```python
from build123d import *

# Parameters (mm, degrees)
SKETCH1_R           = 15
BOSS_EXTRUDE1_DEPTH = 8
BOSS_EXTRUDE2_START = 3
SKETCH2_R           = 16
BOSS_EXTRUDE2_DEPTH = 2
BOSS_EXTRUDE3_START = 3
SKETCH3_R           = 13.5
BOSS_EXTRUDE3_DEPTH = 2
BOSS_EXTRUDE4_START = -1
SKETCH4_R           = 3.6
BOSS_EXTRUDE4_DEPTH = 10
BOSS_EXTRUDE5_START = -1
SKETCH5_R           = 0.9
BOSS_EXTRUDE5_DEPTH = 10
BOSS_EXTRUDE6_START = -1
SKETCH6_R           = 0.9
BOSS_EXTRUDE6_DEPTH = 10
BOSS_EXTRUDE7_START = -1
SKETCH7_R           = 0.9
BOSS_EXTRUDE7_DEPTH = 10
BOSS_EXTRUDE8_START = -1
SKETCH8_R           = 0.9
BOSS_EXTRUDE8_DEPTH = 10


with BuildPart() as part:
    # Sketch1 → Boss-Extrude1 (new body)
    with BuildSketch(Plane(origin=(0, 0, 0), x_dir=(0, 0, -1), z_dir=(1, 0, 0))):
        Circle(SKETCH1_R)
    extrude(amount=BOSS_EXTRUDE1_DEPTH)


with BuildPart() as body_2:
    # Sketch2 → Boss-Extrude2 (new body)
    with BuildSketch(Plane(origin=(0, 0, 0), x_dir=(0, 0, -1), z_dir=(1, 0, 0)).offset(BOSS_EXTRUDE2_START)):
        Circle(SKETCH2_R)
    extrude(amount=BOSS_EXTRUDE2_DEPTH)


with BuildPart() as part_1:
    add(part.part)

    # Combine1: cut body 2
    add(body_2.part, mode=Mode.SUBTRACT)

    # Sketch3 → Boss-Extrude3 (add)
    with BuildSketch(Plane(origin=(0, 0, 0), x_dir=(0, 0, -1), z_dir=(1, 0, 0)).offset(BOSS_EXTRUDE3_START)):
        Circle(SKETCH3_R)
    extrude(amount=BOSS_EXTRUDE3_DEPTH)


with BuildPart() as body_2_2:
    # Sketch4 → Boss-Extrude4 (new body)
    with BuildSketch(Plane(origin=(0, 0, 0), x_dir=(0, 0, -1), z_dir=(1, 0, 0)).offset(BOSS_EXTRUDE4_START)):
        Circle(SKETCH4_R)
    extrude(amount=BOSS_EXTRUDE4_DEPTH)


with BuildPart() as part_2:
    add(part_1.part)

    # Combine2: cut body 2 2
    add(body_2_2.part, mode=Mode.SUBTRACT)


with BuildPart() as body_2_3:
    # Sketch5 → Boss-Extrude5 (new body)
    with BuildSketch(Plane(origin=(0, 0, 0), x_dir=(0, 0, -1), z_dir=(1, 0, 0)).offset(BOSS_EXTRUDE5_START)):
        with Locations((0, -10)):
            Circle(SKETCH5_R)
    extrude(amount=BOSS_EXTRUDE5_DEPTH)


with BuildPart() as part_3:
    add(part_2.part)

    # Combine3: cut body 2 3
    add(body_2_3.part, mode=Mode.SUBTRACT)


with BuildPart() as body_2_4:
    # Sketch6 → Boss-Extrude6 (new body)
    with BuildSketch(Plane(origin=(0, 0, 0), x_dir=(0, 0, -1), z_dir=(1, 0, 0)).offset(BOSS_EXTRUDE6_START)):
        with Locations((0, -7)):
            Circle(SKETCH6_R)
    extrude(amount=BOSS_EXTRUDE6_DEPTH)


with BuildPart() as part_4:
    add(part_3.part)

    # Combine4: cut body 2 4
    add(body_2_4.part, mode=Mode.SUBTRACT)


with BuildPart() as body_2_5:
    # Sketch7 → Boss-Extrude7 (new body)
    with BuildSketch(Plane(origin=(0, 0, 0), x_dir=(0, 0, -1), z_dir=(1, 0, 0)).offset(BOSS_EXTRUDE7_START)):
        with Locations((0, 7)):
            Circle(SKETCH7_R)
    extrude(amount=BOSS_EXTRUDE7_DEPTH)


with BuildPart() as part_5:
    add(part_4.part)

    # Combine5: cut body 2 5
    add(body_2_5.part, mode=Mode.SUBTRACT)


with BuildPart() as body_2_6:
    # Sketch8 → Boss-Extrude8 (new body)
    with BuildSketch(Plane(origin=(0, 0, 0), x_dir=(0, 0, -1), z_dir=(1, 0, 0)).offset(BOSS_EXTRUDE8_START)):
        with Locations((0, 10)):
            Circle(SKETCH8_R)
    extrude(amount=BOSS_EXTRUDE8_DEPTH)


with BuildPart() as part_6:
    add(part_5.part)

    # Combine6: cut body 2 6
    add(body_2_6.part, mode=Mode.SUBTRACT)


solid = part_6.part
```
Input: part model. Units: mm. Frame: model coordinates. A direction names the side the tool comes from. Round coordinates to 2 decimals unless told otherwise and drop trailing zeros. Loops run counter-clockwise (first coordinate to the right, second up) from the corner with the lowest first, then second, coordinate; pieces in that order, holes last. Notation, with made-up numbers: (80, 31) -> (101, 31) arc R10 cw to (101, 38) -> close; hole circle Ø9 at (56.25, -25). An arc over 180 degrees is marked (long way). Use one line per item in the form item = value. Start each with the question number.
Item 1: Contact query for flat-ended pins moving along their axis: pin 1 Ø3 at (x, y) = (4, 10.5) entering from -Z; pin 2 Ø2 at (x, z) = (5.5, -7.5) entering from +Y; pin 3 Ø2 at (x, z) = (7, -1.5) entering from -Y. Output: stop coordinate, or through.
Item 2: Mould query, pull axis Z, two halves, no side actions, for faces 1 (the face through (3.94, -6.11, 0.12)), 2 (the face through (8, -3, -3)), 3 (the face through (6.479, 0.66, 14.985)). Classes: pulls with the +Z half, pulls with the -Z half, needs draft (parallel to the pull), parting line crosses it, or undercut.
Item 3: Section query D-D on z = -9. Return the cut outline in (x, y).
Item 4: Set-up query: faces 4 (the face through (3.94, 10.89, 0.12)), 5 (the face through (3.99, -13.18, 2.93)). Return all of +Z, -Z, +X, -X, +Y, -Y with unobstructed straight access to the full face (end or side cutting, diameter ignored); none if empty.
Item 5: Section query C-C on x = 4.5. Return the cut outline in (y, z), then the cut area to 3 significant figures.
Item 6: Section query A-A on z = 0. Count the separate pieces of the cut face and the enclosed holes in it, then the cut area to 3 significant figures.
Item 7: Section query B-B on y = 10. Return the cut outline in (x, z).
Item 8: Material intervals for L1, parallel to Y at x = 6.25, z = 0; L2, parallel to Y at x = 4.5, z = 0; L3, parallel to X at y = -0.25, z = -14, sorted ascending. Write a range as from..to.
Ans:
q1.pin_1 = -11.7
q1.pin_2 = 13.52
q1.pin_3 = -14.99
q2.face_1 = undercut
q2.face_2 = needs draft
q2.face_3 = parting line crosses it
q3.outline = (0, -12) -> (3, -12) -> (3, -10.06) -> (5, -10.06) -> (5, -12) -> (8, -12) -> (8, 12) -> (5, 12) -> (5, 10.06) -> (3, 10.06) -> (3, 12) -> (0, 12) -> close
q4.face_4 = +X, -X
q4.face_5 = none
q5.outline = circle Ø27 at (0, 0); hole circle Ø1.8 at (-10, 0); hole circle Ø1.8 at (-7, 0); hole circle Ø7.2 at (0, 0); hole circle Ø1.8 at (7, 0); hole circle Ø1.8 at (10, 0)
q5.area = 522 mm^2
q6.separate_pieces = 6
q6.enclosed_holes = 0
q6.area = 119 mm^2
q7.outline = (0, -11.18) -> (3, -11.18) -> (3, -9.07) -> (5, -9.07) -> (5, -11.18) -> (8, -11.18) -> (8, -0.9) -> (0, -0.9) -> close; (0, 0.9) -> (8, 0.9) -> (8, 11.18) -> (5, 11.18) -> (5, 9.07) -> (3, 9.07) -> (3, 11.18) -> (0, 11.18) -> close
q8.L1 = -15..-10.9, -9.1..-7.9, -6.1..-3.6, 3.6..6.1, 7.9..9.1, 10.9..15
q8.L2 = -13.5..-10.9, -9.1..-7.9, -6.1..-3.6, 3.6..6.1, 7.9..9.1, 10.9..13.5
q8.L3 = 0..3, 5..8
